from build123d import *

# Parameters (mm, degrees)
F1_DEPTH       = 25
F2_R           = 18
F3_DEPTH       = 18
F4_R           = 15.4
F5_DEPTH       = 7
F6_R           = 5
F7_DEPTH       = 25
F9_DEPTH       = 22
F11_END_RADIUS = 18
F11_REACH      = 68.8481644957


with BuildPart() as f1:
    # F0 (on Front) → F1 (new body)
    with BuildSketch(Plane.XZ):
        with BuildLine():
            Line((60, 11), (60, 23.5))
            Line((60, 23.5), (60, 36))
            Line((60, 36), (31.0034618727, 45.7698913317))
            ThreePointArc((31.0034618727, 45.7698913317), (0, 23.5), (31.0034618727, 1.2301086683))
            Line((31.0034618727, 1.2301086683), (60, 11))
        make_face()
    extrude(amount=F1_DEPTH)

    # F2 (on face) → F3 (cut)
    with BuildSketch(Plane.XZ.offset(25)):
        with Locations((23.5, 23.5)):
            Circle(F2_R)
    extrude(amount=-F3_DEPTH, mode=Mode.SUBTRACT)

    # F4 (on face) → F5 (cut)
    with BuildSketch(Plane(origin=(0, 0, 0), x_dir=(-1, 0, 0), z_dir=(0, 1, 0))):
        with Locations((-23.5, 23.5)):
            Circle(F4_R)
    extrude(amount=-F5_DEPTH, mode=Mode.SUBTRACT)

    # F6 (on face) → F7 (cut)
    with BuildSketch(Plane.YZ.offset(60)):
        with Locations((-15, 23.5)):
            Circle(F6_R)
    extrude(amount=-F7_DEPTH, mode=Mode.SUBTRACT)

    # F8 (on face) → F9 (cut)
    with BuildSketch(Plane.XZ.offset(25)):
        with BuildLine():
            Line((52, 16), (52, 23.5))
            Line((52, 23.5), (52, 31))
            Line((52, 31), (39.863068172, 31))
            ThreePointArc((39.863068172, 31), (41.0860061852, 27.3382791004), (41.5, 23.5))
            ThreePointArc((41.5, 23.5), (41.0860061852, 19.6617208996), (39.863068172, 16))
            Line((39.863068172, 16), (52, 16))
        make_face()
    extrude(amount=-F9_DEPTH, mode=Mode.SUBTRACT)

    f11_end = (Plane(origin=(23.5, -5, 23.5), x_dir=(0, 0, -1), z_dir=(0, -1, 0)) * Cylinder(F11_END_RADIUS, 298.1207660327, mode=Mode.PRIVATE)).faces().sort_by_distance((41.5, -5, 23.5))[0]
    # F10 (on face) → F11 (join, up to the whole of a round face its end follows)
    with BuildSketch(Plane(origin=(52, 0, 0), x_dir=(0, -1, 0), z_dir=(-1, 0, 0))):
        Polygon((3, 16), (10.6698729811, 16), (6.3397459622, 23.5), (10.6698729811, 31), (3, 31), align=None)
    f11_long = extrude(amount=F11_REACH, mode=Mode.PRIVATE)
    add(split(f11_long, bisect_by=f11_end, keep=Keep.ALL, mode=Mode.PRIVATE).solids().sort_by_distance((52, -5.8943260873, 23.5))[0])


solid = f1.part
The listing builds one solid part. Answer for the finished solid, in the listing's coordinates (mm). A direction names the side the tool comes from. Coordinates: 2 decimals unless noted, no trailing zeros. Loops run counter-clockwise (first coordinate to the right, second up) from the corner with the lowest first, then second, coordinate; pieces in that order, holes last. Notation, with made-up numbers: M -33.75,-34 L -10.75,-34 A11 ccw -10.75,-30 Z; hole C 71.5,38 d3. An arc over 180 degrees is marked long. Answer in a Markdown table with one row per item.
1) Determine the mould class of faces 1 (the cylindrical face through (56.06, -16.08, 18.62)), 2 (the flat face through (46, -18, 31)), 3 (the flat face through (46.016, -8.535, 19.697)) for opening direction Y: released by +Y, released by -Y, zero draft, split by the parting line, or undercut.
Answers below:
| item | result |
|---|---|
| face 1 | undercut |
| face 2 | zero draft |
| face 3 | released by -Y |
2) Find section B-B (x = 23.5). Determine the outline of the cut face in (y, z).
Answers below:
| item | result |
|---|---|
| outline | M -25,0 L 0,0 L 0,8.1 L -7,8.1 L -7,5.5 L -25,5.5 Z; M -25,41.5 L -7,41.5 L -7,38.9 L 0,38.9 L 0,47 L -25,47 Z |
3) Given pin 1 (13.5 mm diameter, centred on x = 46.5, y = -18, fed in from -Z); pin 2 (2 mm diameter, centred on x = 32, y = -7, fed in from +Z); pin 3 (9.5 mm diameter, centred on x = 43.5, y = -16.5, fed in from +Z), each flat-ended and moving along its own axis, determine where each tip first touches the part or whether it passes through.
Answers below:
| item | result |
|---|---|
| pin 1 | z = 4.18 |
| pin 2 | z = 45.77 |
| pin 3 | z = 43.16 |
4) Find section C-C (y = -15). Determine the outline of the cut face in (x, z).
Answers below:
| item | result |
|---|---|
| outline | M 31,1.23 L 60,11 L 60,18.5 L 52,18.5 L 52,16 L 39.86,16 A18 cw long 39.86,31 L 52,31 L 52,28.5 L 60,28.5 L 60,36 L 31,45.77 A23.5 ccw long Z |
5) Find section D-D (y = -9). Determine the outline of the cut face in (x, z).
Answers below:
| item | result |
|---|---|
| outline | M 31,1.23 L 60,11 L 60,36 L 31,45.77 A23.5 ccw long Z; hole M 40.9,18.89 L 52,18.89 L 52,28.11 L 40.9,28.11 A18 ccw long Z |
6) Find the intervals of material crossed by probe 1 along Z at (x, y) = (23.5, -2); probe 2 along Z at (x, y) = (23.5, -18); probe 3 along X at (y, z) = (-5.75, 20.5), in increasing order.
Answers below:
| item | result |
|---|---|
| probe 1 | 0 to 8.1, 38.9 to 47 |
| probe 2 | 0 to 5.5, 41.5 to 47 |
| probe 3 | 0.19 to 8.4, 38.6 to 60 |
7) Find section A-A (y = -22.5). Determine the outline of the cut face in (x, z), then the cut area to 3 significant figures.
Answers below:
| item | result |
|---|---|
| outline | M 31,1.23 L 60,11 L 60,36 L 31,45.77 A23.5 ccw long Z; hole M 39.86,16 L 52,16 L 52,31 L 39.86,31 A18 ccw long Z |
| area | 1,040 mm^2 |
8) Which of the six approach directions +Z, -Z, +X, -X, +Y, -Y give full straight-line access (tool end or side, diameter ignored) to faces 4 (the flat face through (45.299, -12.325, 6.047)), 5 (the flat face through (46.016, -8.474, 27.198))?
Answers below:
| item | result |
|---|---|
| face 4 | -Z, +X, +Y, -Y |
| face 5 | -Y |
